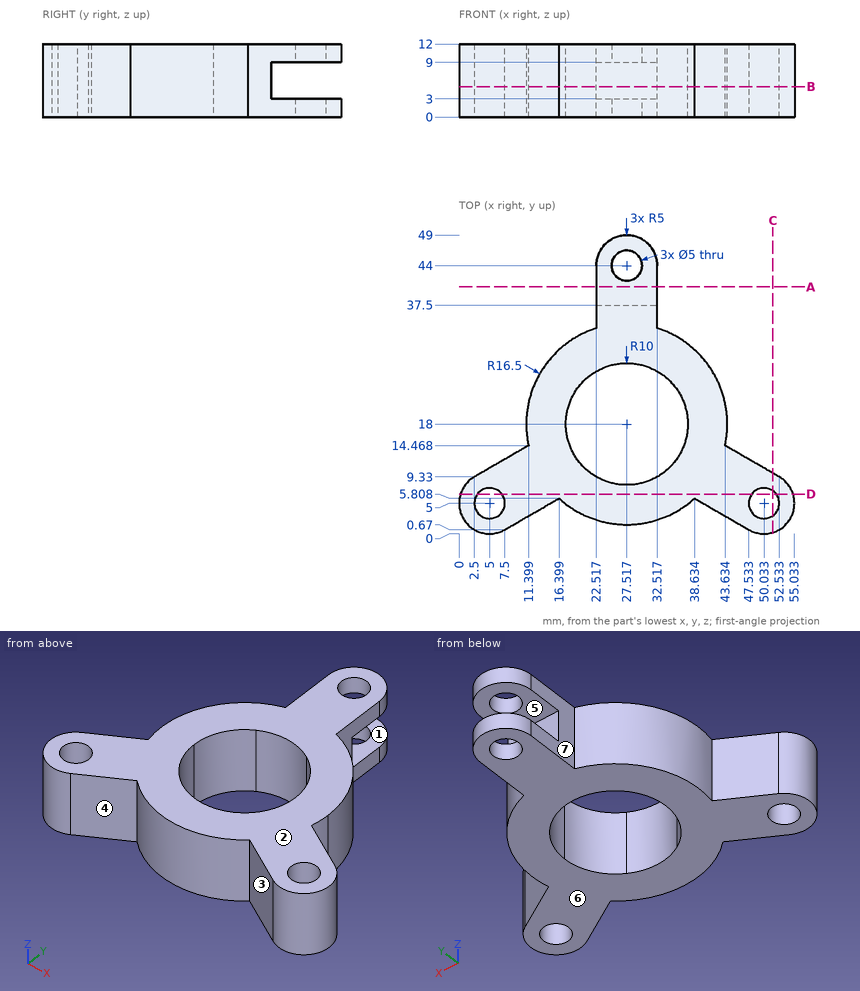
The drawing under review shows one solid part. Ordinate dimensions are in mm from its lowest x, y, z. A direction names the side the tool comes from. Coordinates: 2 decimals unless noted, no trailing zeros. Loops run counter-clockwise (first coordinate to the right, second up) from the corner with the lowest first, then second, coordinate; pieces in that order, holes last. Notation, with made-up numbers: (-36, 65.25) -> (-31, 65.25) arc R18 cw to (-31, 97.25) -> close; hole circle Ø1 at (-28.75, 54.25). An arc over 180 degrees is marked (long way). Answer as a JSON object with one key per item and string values.
Q1. Take a section at A-A on y = 40.5. Give the boundary of the cut face in (x, z).
Answer block:
{"outline": "(22.52, 0) -> (32.52, 0) -> (32.52, 3) -> (22.52, 3) -> close; (22.52, 9) -> (32.52, 9) -> (32.52, 12) -> (22.52, 12) -> close"}
Q2. Take a section at B-B on z = 5. Give the boundary of the cut face in (x, y), plus the area to 3 significant figures.
Answer block:
{"outline": "(2.5, 9.33) arc R5 ccw to (7.5, 0.67) -> (16.4, 5.81) arc R16.5 ccw to (38.63, 5.81) -> (47.53, 0.67) arc R5 ccw to (52.53, 9.33) -> (43.63, 14.47) arc R16.5 ccw to (32.52, 33.72) -> (32.52, 37.5) -> (22.52, 37.5) -> (22.52, 33.72) arc R16.5 ccw to (11.4, 14.47) -> close; hole circle Ø5 at (5, 5); hole circle Ø20 at (27.52, 18); hole circle Ø5 at (50.03, 5)", "area": "808 mm^2"}
Q3. The part is to be moulded in two halves that separate along Z. For the marked faces 1, 2 and 3, say which applies: +Z half, -Z half, draft (parallel to the pull), parting line (faces both ways), or undercut.
Answer block:
{"face 1": "undercut", "face 2": "+Z half", "face 3": "draft"}
Q4. Clearance check with flat-ended pins moving along their axes: pin 1 Ø3 at (x, y) = (27.52, 44) entering from +Z (1 decimal); pin 2 Ø5 at (y, z) = (28.5, 5.5) entering from +X; pin 3 Ø2 at (y, z) = (39, 2) entering from +X; pin 4 Ø2 at (y, z) = (9, 3) entering from -X. State where each tip first meets the part, or that it passes through.
Answer block:
{"pin 1": "passes through", "pin 2": "stops at x = 41.95", "pin 3": "stops at x = 32.52", "pin 4": "stops at x = 1"}
Q5. Tool access review of the marked faces 4, 5, 6 and 7: name each direction out of +Z, -Z, +X, -X, +Y, -Y from which nothing blocks a thin tool from reaching the whole face with its end or side.
Answer block:
{"face 4": "+Z, -Z, -Y", "face 5": "+X, -X, +Y", "face 6": "-Z, +X, -X, +Y, -Y", "face 7": "+Z, -Z, -X, +Y"}
Q6. Take a section at C-C on x = 51.5. Give the boundary of the cut face in (y, z) (1 decimal), plus the area to 3 significant figures.
Answer block:
{"outline": "(0.2, 0) -> (3, 0) -> (3, 12) -> (0.2, 12) -> close; (7, 0) -> (9.9, 0) -> (9.9, 12) -> (7, 12) -> close", "area": "67.9 mm^2"}
Q7. To check wall thickness, follow L1, parallel to X at y = 6, z = 1 (1 decimal); L2, parallel to X at y = 34, z = 8.5; L3, parallel to Y at x = 31, z = 4. State the ranges of each line that lie inside material, in increasing order.
Answer block:
{"L1": "x = 0.1 to 2.7, 7.3 to 47.7, 52.3 to 54.9", "L2": "x = 22.52 to 32.52", "L3": "y = 1.87 to 8.63, 27.37 to 37.5"}
Q8. Take a section at D-D on y = 6.5. Give the boundary of the cut face in (x, z), plus the area to 3 significant figures.
Answer block:
{"outline": "(0.23, 0) -> (3, 0) -> (3, 12) -> (0.23, 12) -> close; (7, 0) -> (48.03, 0) -> (48.03, 12) -> (7, 12) -> close; (52.03, 0) -> (54.8, 0) -> (54.8, 12) -> (52.03, 12) -> close", "area": "559 mm^2"}
